Here's the drawing with two shaded views (mm, measured from the low corner). I have some questions. Round coordinates to 2 decimals unless told otherwise and drop trailing zeros. Order: outer loops, then holes, each group sorted by start corner. A loop starts at its lowest first (then second) coordinate and runs counter-clockwise, first axis right, second up. Notation, with made-up numbers: (-11, 36.5) -> (45, 36.5) arc R16 ccw to (45, 54.5) -> close; hole circle Ø3 at (44.25, 39.25). An arc over 180 degrees is marked (long way). Use a Markdown table: item, result. Add a question column.
Q1. I'm going to push flat-ended pins straight in: pin 1 Ø3.5 at (x, z) = (47, 105) entering from +Y; pin 2 Ø7 at (x, z) = (78.57, 78.57) entering from +Y. Where does each tip first touch, or does it pass through?
Q2. If we section it at D-D on y = 2.2: Give the number of separate pieces and of enclosed holes in the cut face, plus the area to 3 significant figures.
Q3. If we section it at A-A on z = 78.57: List the corners of the cut face in (x, y) for me.
Q4. If we section it at B-B on x = 31.43: List the corners of the cut face in (y, z) for me, plus the area to 3 significant figures.
Q5. I need wall thicknesses on line 1 along Z through (x, y) = (78.57, 1); line 2 along Z through (x, y) = (6, 3.45); line 3 along X through (y, z) = (2.65, 105). Which ranges of each line are inside material? Lowest first, please. Write a range as [from, to].
Q6. We'd pull the mould along Z, two halves only. Please class the marked faces 1 and 2: +Z half, -Z half, draft (parallel to the pull), parting line (faces both ways), or undercut.
Q7. If we section it at C-C on x = 55: List the corners of the cut face in (y, z) for me, plus the area to 4 significant figures.
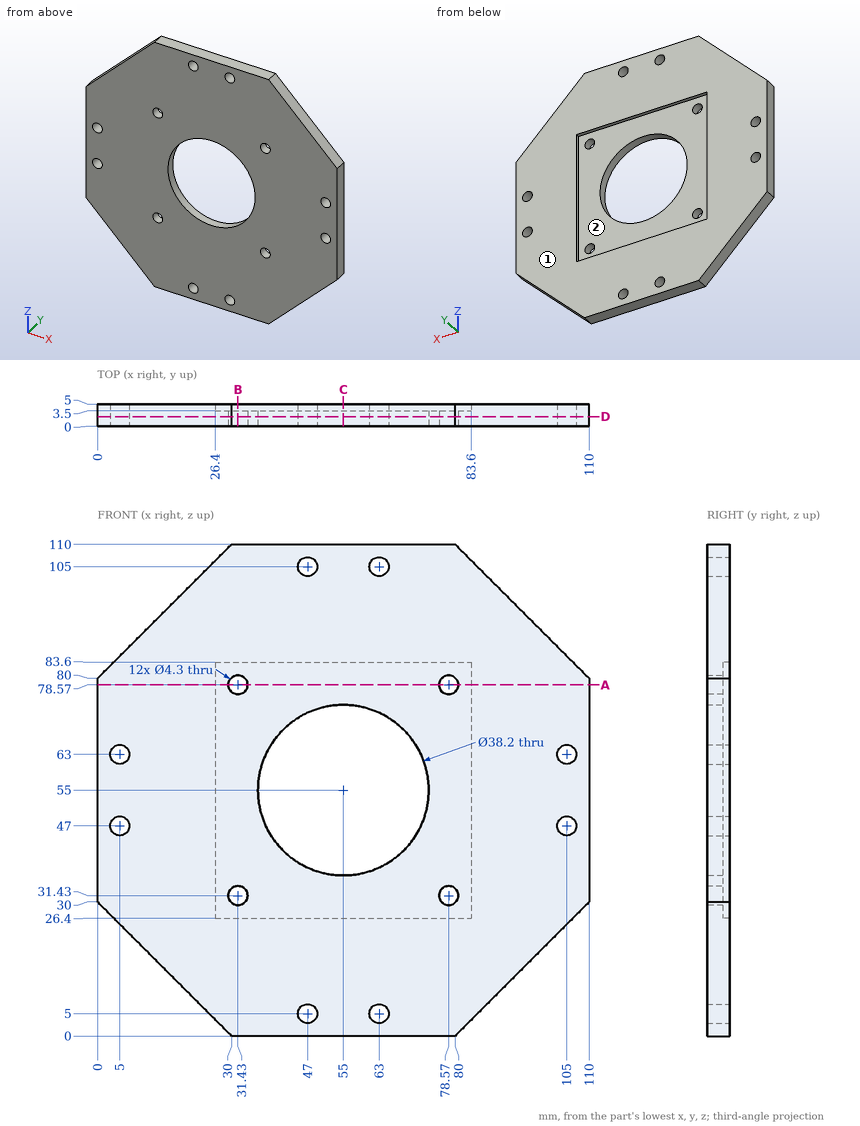
Answer below:
| question | item | result |
|---|---|---|
| 1 | pin 1 | through |
| 1 | pin 2 | y = 3.5 |
| 2 | separate pieces | 1 |
| 2 | enclosed holes | 13 |
| 2 | area | 8,980 mm² |
| 3 | outline | (0, 0) -> (29.28, 0) -> (29.28, 3.5) -> (26.4, 3.5) -> (26.4, 5) -> (0, 5) -> close; (33.58, 0) -> (76.42, 0) -> (76.42, 3.5) -> (33.58, 3.5) -> close; (80.72, 0) -> (110, 0) -> (110, 5) -> (83.6, 5) -> (83.6, 3.5) -> (80.72, 3.5) -> close |
| 4 | outline | (0, 0) -> (5, 0) -> (5, 26.4) -> (3.5, 26.4) -> (3.5, 29.28) -> (0, 29.28) -> close; (0, 33.58) -> (3.5, 33.58) -> (3.5, 76.42) -> (0, 76.42) -> close; (0, 80.72) -> (3.5, 80.72) -> (3.5, 83.6) -> (5, 83.6) -> (5, 110) -> (0, 110) -> close |
| 4 | area | 434 mm² |
| 5 | line 1 | [0, 29.28], [33.58, 76.42], [80.72, 110] |
| 5 | line 2 | [24, 45.1], [48.9, 61.1], [64.9, 86] |
| 5 | line 3 | [25, 44.85], [49.15, 60.85], [65.15, 85] |
| 6 | face 1 | draft |
| 6 | face 2 | undercut |
| 7 | outline | (0, 0) -> (5, 0) -> (5, 26.4) -> (3.5, 26.4) -> (3.5, 35.9) -> (0, 35.9) -> close; (0, 74.1) -> (3.5, 74.1) -> (3.5, 83.6) -> (5, 83.6) -> (5, 110) -> (0, 110) -> close |
| 7 | area | 330.5 mm² |
